Could you check a few things on this model? Use its own coordinates, in mm. Coordinates: 2 decimals unless noted, no trailing zeros. Order: outer loops, then holes, each group sorted by start corner. A loop starts at its lowest first (then second) coordinate and runs counter-clockwise, first axis right, second up. Notation, with made-up numbers: (73.25, 59) -> (110.25, 59) arc R32 ccw to (110.25, 98) -> close; hole circle Ø5 at (67, -27.75). An arc over 180 degrees is marked (long way). Put each result on its own line as item: value. Start each with the question number.
Q1. If we section it at B-B (x = 0): Please give me the cut outline in (y, z), and give its area (3 significant figures).
Q2. Will these pins go through, and if not, where does the flat tip stop? pin 1 (4 mm diameter, centred on x = 0, z = 0, fed in from -Y); pin 2 (1 mm diameter, centred on x = 3.5, z = -5, fed in from -Y); pin 3 (18.5 mm diameter, centred on y = -19.939, z = 0, fed in from +X).
Q3. Please list where these lines run through material, in increasing order: line 1 along X through (y, z) = (-8, 0); line 2 along Z through (x, y) = (0, -9.75); line 3 along X through (y, z) = (-11.5, 0).
Q4. If we section it at A-A (z = 0): Please give me the cut outline in (x, y), and give its area (3 significant figures).
Q5. If we section it at C-C (x = -80): Please give me the cut outline in (y, z), and give its area (3 significant figures).
from build123d import *

# Parameters (mm, degrees)
F1_DEPTH = 39.878
F2_R     = 5.767295
F3_DEPTH = 279.401
F4_R     = 5.08


with BuildPart() as f1:
    # F0 (on Front) → F1 (new body)
    with BuildSketch(Plane.XZ):
        with BuildLine():
            Line((139.7, 0), (139.7, 19.939))
            Line((139.7, 19.939), (-139.7, 19.939))
            Line((-139.7, 19.939), (-139.7, 0))
            Line((-139.7, 0), (-2.4892, 0))
            ThreePointArc((-2.4892, 0), (0, 2.4892), (2.4892, 0))
            Line((2.4892, 0), (139.7, 0))
        make_face()
        with BuildLine():
            Line((139.7, -19.939), (139.7, 0))
            Line((139.7, 0), (2.4892, 0))
            ThreePointArc((2.4892, 0), (0, -2.4892), (-2.4892, 0))
            Line((-2.4892, 0), (-139.7, 0))
            Line((-139.7, 0), (-139.7, -19.939))
            Line((-139.7, -19.939), (139.7, -19.939))
        make_face()
    extrude(amount=F1_DEPTH)

    # F2 (on face) → F3 (cut, through all)
    with BuildSketch(Plane.YZ.offset(139.7)):
        with Locations((-19.939, 0)):
            Circle(F2_R)
    extrude(amount=-F3_DEPTH, mode=Mode.SUBTRACT)

    # F4
    f4_edges = [f1.edges().sort_by_distance(p)[0] for p in [
        (139.7, -25.706295, 0),
        (-2.4892, -39.878, 0),
        (0, -39.878, 19.939),
        (0, 0, 19.939),
        (0, 0, -19.939),
        (0, -39.878, -19.939),
    ]]
    fillet(f4_edges, radius=F4_R)


solid = f1.part
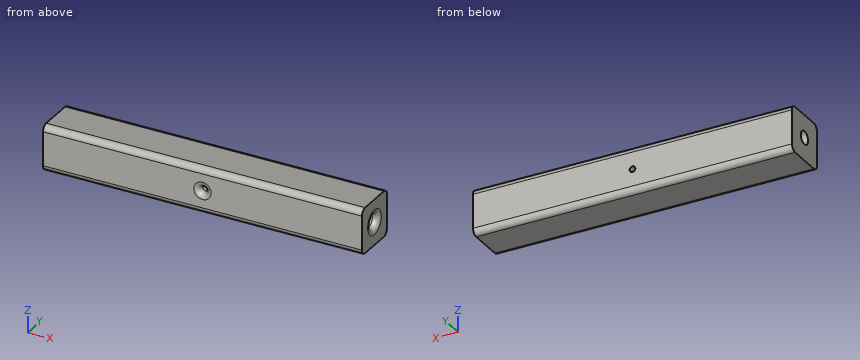
The answers:
1. outline: (-39.88, -14.86) arc R5.08 ccw to (-34.8, -19.94) -> (-5.08, -19.94) arc R5.08 ccw to (0, -14.86) -> (0, -2.49) -> (-14.74, -2.49) arc R5.77 cw to (-25.14, -2.49) -> (-34.8, -2.49) arc R5.08 ccw to (-39.88, -7.57) -> close; (-39.88, 7.57) arc R5.08 ccw to (-34.8, 2.49) -> (-25.14, 2.49) arc R5.77 cw to (-14.74, 2.49) -> (0, 2.49) -> (0, 14.86) arc R5.08 ccw to (-5.08, 19.94) -> (-34.8, 19.94) arc R5.08 ccw to (-39.88, 14.86) -> close
1. area: 1,310 mm^2
2. pin 1: through
2. pin 2: y = -39.79
2. pin 3: x = 139.44
3. line 1: -139.7 to -2.49, 2.49 to 139.7
3. line 2: -19.94 to -2.49, 2.49 to 19.94
3. line 3: -139.7 to -2.49, 2.49 to 139.09
4. outline: (-139.7, -39.88) -> (-7.57, -39.88) arc R5.08 ccw to (-2.49, -34.8) -> (-2.49, -25.71) -> (-139.7, -25.71) -> close; (-139.7, -14.17) -> (-2.49, -14.17) -> (-2.49, 0) -> (-139.7, 0) -> close; (2.49, -34.8) arc R5.08 ccw to (7.57, -39.88) -> (139.7, -39.88) -> (139.7, -30.79) arc R5.08 ccw to (134.62, -25.71) -> (2.49, -25.71) -> close; (2.49, -14.17) -> (134.62, -14.17) arc R5.08 ccw to (139.7, -9.09) -> (139.7, 0) -> (2.49, 0) -> close
4. area: 7,760 mm^2
5. outline: (-39.88, -14.86) arc R5.08 ccw to (-34.8, -19.94) -> (-5.08, -19.94) arc R5.08 ccw to (0, -14.86) -> (0, 14.86) arc R5.08 ccw to (-5.08, 19.94) -> (-34.8, 19.94) arc R5.08 ccw to (-39.88, 14.86) -> close; hole circle Ø11.53 at (-19.94, 0)
5. area: 1,460 mm^2
